from build123d import *

# Parameters (mm, degrees)
SKETCH1_R               = 10
BOSS_EXTRUDE1_DEPTH     = 21
BOSS_EXTRUDE2_DEPTH     = 3
SKETCH3_R               = 7
BOSS_EXTRUDE3_DEPTH     = 6
SKETCH4_R               = 6
CUT_EXTRUDE1_DEPTH      = 25
SKETCH5_R               = 4
CUT_EXTRUDE2_DEPTH      = 2
CUT_EXTRUDE3_REACH      = 34.276
CUT_EXTRUDE3_END_RADIUS = 6
SKETCH5_3_R             = 2.5
SKETCH6_R               = 1.55
CUT_EXTRUDE4_DEPTH      = 27.931170886


with BuildPart() as part:
    # Sketch1 → Boss-Extrude1 (new body)
    with BuildSketch(Plane(origin=(0, 0, 0), x_dir=(1, 0, 0), z_dir=(0, 1, 0))):
        with Locations(Location((0, 0, 0), (0, 0, 90))):
            Circle(SKETCH1_R)
    extrude(amount=BOSS_EXTRUDE1_DEPTH)

    # Sketch2 → Boss-Extrude2 (add)
    with BuildSketch(Plane.XZ):
        with BuildLine():
            Line((-7.985787442, 12.928156025), (7.985787442, 12.928156025))
            ThreePointArc((7.985787442, 12.928156025), (10.823619675, 0.815257434), (7.985787442, -11.297641157))
            Line((7.985787442, -11.297641157), (-7.985787442, -11.297641157))
            ThreePointArc((-7.985787442, -11.297641157), (-10.823619675, 0.815257434), (-7.985787442, 12.928156025))
        make_face()
    extrude(amount=BOSS_EXTRUDE2_DEPTH)

    # Sketch3 → Boss-Extrude3 (add)
    with BuildSketch(Plane.XZ.offset(3)):
        with Locations(Location((0, 0, 0), (0, 0, 270))):
            Circle(SKETCH3_R)
    extrude(amount=BOSS_EXTRUDE3_DEPTH)

    # Sketch4 → Cut-Extrude1 (cut)
    with BuildSketch(Plane.XZ.offset(9)):
        with Locations(Location((0, 0, 0), (0, 0, 270))):
            Circle(SKETCH4_R)
    extrude(amount=-CUT_EXTRUDE1_DEPTH, mode=Mode.SUBTRACT)

    # Sketch5 → Cut-Extrude2 (cut)
    with BuildSketch(Plane(origin=(10, 0, 0), x_dir=(0, 0, -1), z_dir=(1, 0, 0))):
        with Locations((0, 11)):
            Circle(SKETCH5_R)
    extrude(amount=-CUT_EXTRUDE2_DEPTH, mode=Mode.SUBTRACT)

    # Cut-Extrude3: up to this cylinder (the profile starts outside it)
    cut_extrude3_end = Plane(origin=(0, 11, 0), z_dir=(0, -1, 0)) * Cylinder(CUT_EXTRUDE3_END_RADIUS, 81.552, mode=Mode.PRIVATE)
    # Sketch5<3> → Cut-Extrude3 (cut, up to the surface)
    with BuildSketch(Plane(origin=(10, 0, 0), x_dir=(0, 0, -1), z_dir=(1, 0, 0)), mode=Mode.PRIVATE) as cut_extrude3_sk1:
        with Locations((0, 11)):
            Circle(SKETCH5_3_R)
    cut_extrude3_tool1 = extrude(cut_extrude3_sk1.sketch, amount=-CUT_EXTRUDE3_REACH, mode=Mode.PRIVATE) - cut_extrude3_end
    add(cut_extrude3_tool1.solids().sort_by_distance((10, 11, 0))[0], mode=Mode.SUBTRACT)

    # Sketch6 → Cut-Extrude4 (cut, through all)
    with BuildSketch(Plane(origin=(0, 0, 0), x_dir=(1, 0, 0), z_dir=(0, 1, 0))):
        with Locations((0.39625422, 13.700444465)):
            Circle(SKETCH6_R)
        with Locations((-0.346325383, -13.735993833)):
            Circle(SKETCH6_R)
    extrude(amount=-CUT_EXTRUDE4_DEPTH, mode=Mode.SUBTRACT)


solid = part.part
The listing builds one solid part. Answer for the finished solid, in the listing's coordinates (mm). A direction names the side the tool comes from. Coordinates: 2 decimals unless noted, no trailing zeros. Loops run counter-clockwise (first coordinate to the right, second up) from the corner with the lowest first, then second, coordinate; pieces in that order, holes last. Notation, with made-up numbers: (74.25, 1.5) -> (86.25, 1.5) arc R13 cw to (86.25, 11.5) -> close; hole circle Ø6 at (-16.5, 58.25). An arc over 180 degrees is marked (long way). Answer in a Markdown table with one row per item. Add a question column.
1. The part is cut by section D-D, the plane y = 16.5. Write down the section's boundary in (x, z), then the cut area to 3 significant figures.
2. For faces 1 (the flat face through (2, 0, 10)), 2 (the flat face through (0, 16, 0)), 3 (the cylindrical face through (6.74, 10.04, -2.31)), determine the directions among +Z, -Z, +X, -X, +Y, -Y from which every point of the face is accessible in a straight line to the end or side of a thin tool.
3. The part is cut by section A-A, the plane z = 0. Write down the section's boundary in (x, y), then the cut area to 3 significant figures.
4. Consider line 1 (Y direction, x = 6.2, z = 0); line 2 (X direction, y = -3.5, z = 0); line 3 (Y direction, x = 7.4, z = 0). Determine where each line is inside the solid, lowest interval first. Write a range as [from, to].
5. The part is cut by section B-B, the plane y = -5.5. Write down the section's boundary in (x, z), then the cut area to 3 significant figures.
6. Determine the mould class of faces 4 (the cylindrical face through (8.792, 9.468, -3.695)), 5 (the flat face through (4, -1, 12.928)), 6 (the flat face through (2, -9, -6)) for opening direction Y: +Y half, -Y half, draft (parallel to the pull), parting line (faces both ways), or undercut.
7. The part is cut by section C-C, the plane x = -2.25. Write down the section's boundary in (y, z), then the cut area to 3 significant figures.
8. Flat-ended cylindrical pins translate along their axes: P1, Ø13, axis at y = 11, z = 0, coming from the -X side; P2, Ø6, axis at y = -4, z = -1.5, coming from the +X side; P3, Ø12, axis at y = 10, z = -8.5, coming from the -X side; P4, Ø10, axis at x = -8.5, z = 8, coming from the -Y side. Find the tip coordinate at first contact, or state that the pin passes through.
Answer below:
| question | item | result |
|---|---|---|
| 1 | outline | circle Ø20 at (0, 0) |
| 1 | area | 314 mm2 |
| 2 | face 1 | +Y |
| 2 | face 2 | -Y |
| 2 | face 3 | +X |
| 3 | outline | (-10.81, -3) -> (-7, -3) -> (-7, -9) -> (-6, -9) -> (-6, 16) -> (6, 16) -> (6, 13.5) -> (8, 13.5) -> (8, 15) -> (10, 15) -> (10, 21) -> (-10, 21) -> (-10, 0) -> (-10.81, 0) -> close; (6, -9) -> (7, -9) -> (7, -3) -> (10.81, -3) -> (10.81, 0) -> (10, 0) -> (10, 7) -> (8, 7) -> (8, 8.5) -> (6, 8.5) -> close |
| 3 | area | 243 mm2 |
| 4 | line 1 | [-9, 8.5], [13.5, 21] |
| 4 | line 2 | [-7, -6], [6, 7] |
| 4 | line 3 | [-3, 8.5], [13.5, 21] |
| 5 | outline | circle Ø14 at (0, 0); hole circle Ø12 at (0, 0) |
| 5 | area | 40.8 mm2 |
| 6 | face 4 | undercut |
| 6 | face 5 | draft |
| 6 | face 6 | -Y half |
| 7 | outline | (-9, -6.63) -> (-3, -6.63) -> (-3, -11.3) -> (0, -11.3) -> (0, -9.74) -> (21, -9.74) -> (21, 9.74) -> (0, 9.74) -> (0, 12.93) -> (-3, 12.93) -> (-3, 6.63) -> (-9, 6.63) -> (-9, 5.56) -> (16, 5.56) -> (16, -5.56) -> (-9, -5.56) -> close |
| 7 | area | 283 mm2 |
| 8 | P1 | x = -10 |
| 8 | P2 | x = 10.82 |
| 8 | P3 | x = -9.68 |
| 8 | P4 | y = -9 |
